from build123d import *

# Parameters (mm, degrees)
EXTRUDE_1_DEPTH     = 24
SKETCH_2_R          = 2.5
EXTRUDE_2_DEPTH     = 1.2
SKETCH_3_R          = 2
EXTRUDE_3_DEPTH     = 0.7
SKETCH_5_R          = 1.5
EXTRUDE_5_DEPTH     = 9.3
SKETCH_6_R          = 8.807991622
SKETCH_6_R_2        = 6
CUT_EXTRUDE_1_DEPTH = 15
CUT_EXTRUDE_2_DEPTH = 9.3


with BuildPart() as part:
    # 草图1 → 凸台-拉伸1 (new body)
    with BuildSketch(Plane.XY):
        Polygon((5, 0), (5, 6), (-5, 6), (-5, -6), (5, -6), align=None)
    extrude(amount=EXTRUDE_1_DEPTH)

    # 草图2 → 凸台-拉伸2 (add)
    with BuildSketch(Plane(origin=(0, 0, 0), x_dir=(-1, 0, 0), z_dir=(0, 0, -1))):
        Circle(SKETCH_2_R)
    extrude(amount=EXTRUDE_2_DEPTH)

    # 草图3 → 凸台-拉伸3 (add)
    with BuildSketch(Plane.XY.offset(24)):
        Circle(SKETCH_3_R)
    extrude(amount=EXTRUDE_3_DEPTH)

    # 草图5 → 凸台-拉伸5 (add)
    with BuildSketch(Plane.XY.offset(24.7)):
        Circle(SKETCH_5_R)
    extrude(amount=EXTRUDE_5_DEPTH)

    # 草图6 → 切除-拉伸1 (cut)
    with BuildSketch(Plane(origin=(0, 0, 0), x_dir=(-1, 0, 0), z_dir=(0, 0, -1))):
        Circle(SKETCH_6_R)
        Circle(SKETCH_6_R_2, mode=Mode.SUBTRACT)
    extrude(amount=-CUT_EXTRUDE_1_DEPTH, mode=Mode.SUBTRACT)

    # 草图7 → 切除-拉伸2 (cut)
    with BuildSketch(Plane.XY.offset(34)):
        Polygon((-1, 0), (-1, 3.342262846), (-2.573415309, 3.342262846), (-2.573415309, -2.211230932), (-1, -2.211230932), align=None)
    extrude(amount=-CUT_EXTRUDE_2_DEPTH, mode=Mode.SUBTRACT)


solid = part.part
Input: part model. Units: mm. Frame: model coordinates. A direction names the side the tool comes from. Give positions to 0.01 mm unless a question says otherwise; leave off trailing zeros. Order: outer loops, then holes, each group sorted by start corner. A loop starts at its lowest first (then second) coordinate and runs counter-clockwise, first axis right, second up. Notation, with made-up numbers: M -14.5,12.25 L 8.5,12.25 A14 cw 8.5,26.25 Z; hole C -17.75,49 d4. An arc over 180 degrees is marked long. Answer as a JSON object with one key per item and string values.
1. Reachability of faces 1 (the flat face through (2.2, 0.1, 24)), 2 (the cylindrical face through (0, -6, 7)), 3 (the flat face through (4, 5, 15)) from +Z, -Z, +X, -X, +Y, -Y: full face, straight path, thin tool, end or side. Return the list, or none.
Result sheet:
{"face 1": "+Z", "face 2": "-Z, -Y", "face 3": "-Z, +X, +Y"}
2. First-contact query: P1, Ø0.8, axis at x = 3, y = 4.5, coming from the -Z side; P2, Ø3, axis at x = 2.5, z = 5, coming from the -Y side; P3, Ø3, axis at x = 3.5, z = 7.5, coming from the -Y side; P4, Ø1, axis at x = 3, z = 26, coming from the +Y side. Flat tips, straight axial feed; report the tip coordinate or a pass-through.
Result sheet:
{"P1": "z = 0", "P2": "y = -5.92", "P3": "y = -5.66", "P4": "through"}
3. Cut plane A-A, the plane y = 0. Output: boundary loops of the cut face in (x, z), and give its area (3 significant figures).
Result sheet:
{"outline": "M -5,0 L -2.5,0 L -2.5,-1.2 L 2.5,-1.2 L 2.5,0 L 5,0 L 5,24 L 2,24 L 2,24.7 L 1.5,24.7 L 1.5,34 L -1,34 L -1,24.7 L -2,24.7 L -2,24 L -5,24 Z", "area": "272 mm²"}
4. Cut plane D-D, the plane y = -5. Output: boundary loops of the cut face in (x, z).
Result sheet:
{"outline": "M -5,15 L -3.32,15 L -3.32,0 L 3.32,0 L 3.32,15 L 5,15 L 5,24 L -5,24 Z"}
5. Cut plane B-B, the plane x = 0.75. Output: boundary loops of the cut face in (y, z), and give its area (3 significant figures).
Result sheet:
{"outline": "M -6,15 L -5.95,15 L -5.95,0 L -2.38,0 L -2.38,-1.2 L 2.38,-1.2 L 2.38,0 L 5.95,0 L 5.95,15 L 6,15 L 6,24 L 1.85,24 L 1.85,24.7 L 1.3,24.7 L 1.3,34 L -1.3,34 L -1.3,24.7 L -1.85,24.7 L -1.85,24 L -6,24 Z", "area": "319 mm²"}
6. Ray query, line 1 (Y direction, x = 1, z = 26.5); line 2 (Z direction, x = 4, y = -5); line 3 (Z direction, x = -2.75, y = 1.5). Return the intervals inside material, ascending. Write a range as [from, to].
Result sheet:
{"line 1": "[-1.12, 1.12]", "line 2": "[15, 24]", "line 3": "[0, 24]"}
7. Cut plane C-C, the plane z = 30. Output: boundary loops of the cut face in (x, y), and give its area (3 significant figures).
Result sheet:
{"outline": "M -1,-1.12 A1.5 ccw long -1,1.12 Z", "area": "6.29 mm²"}
